```python
from build123d import *

# Parameters (mm, degrees)
SKETCH1_R           = 3.55
SKETCH1_R_2         = 1.5
BOSS_EXTRUDE1_DEPTH = 3


with BuildPart() as part:
    # Sketch1 → Boss-Extrude1 (new body)
    with BuildSketch(Plane.XY):
        with BuildLine():
            Line((4, 0), (4, 9.527864045))
            ThreePointArc((4, 9.527864045), (6, 14), (4, 18.472135955))
            Line((4, 18.472135955), (4, 49))
            ThreePointArc((4, 49), (0, 53), (-4, 49))
            Line((-4, 49), (-4, 18.472135955))
            ThreePointArc((-4, 18.472135955), (-6, 14), (-4, 9.527864045))
            Line((-4, 9.527864045), (-4, 0))
            ThreePointArc((-4, 0), (0, -4), (4, 0))
        make_face()
        with Locations((0, 14)):
            Circle(SKETCH1_R, mode=Mode.SUBTRACT)
        with Locations((0, 49)):
            Circle(SKETCH1_R_2, mode=Mode.SUBTRACT)
        with BuildLine():
            Line((-1, 0), (-1, 5))
            ThreePointArc((-1, 5), (0, 6), (1, 5))
            Line((1, 5), (1, 0))
            ThreePointArc((1, 0), (0, -1), (-1, 0))
        make_face(mode=Mode.SUBTRACT)
        with BuildLine():
            Line((-1, 28), (-1, 23))
            ThreePointArc((-1, 23), (0, 22), (1, 23))
            Line((1, 23), (1, 28))
            ThreePointArc((1, 28), (0, 29), (-1, 28))
        make_face(mode=Mode.SUBTRACT)
    extrude(amount=BOSS_EXTRUDE1_DEPTH)


solid = part.part
```
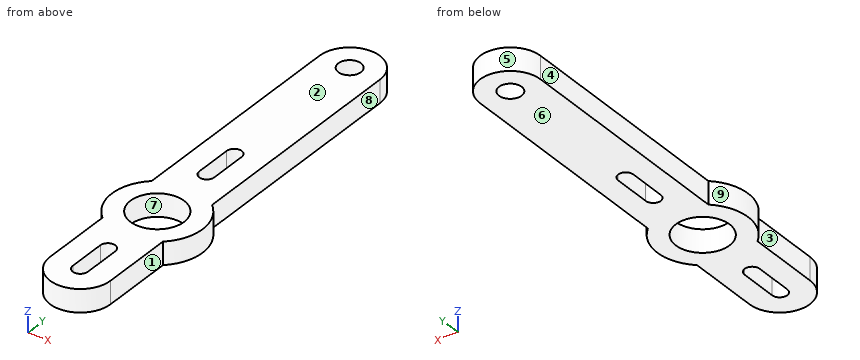
Verification items for the finished model (mm, model axes). Face numbers are marked on the shaded views. A direction names the side the tool comes from. Round coordinates to 2 decimals unless told otherwise and drop trailing zeros. Order: outer loops, then holes, each group sorted by start corner. A loop starts at its lowest first (then second) coordinate and runs counter-clockwise, first axis right, second up.
1) Cross-section at A-A, the plane y = 24. Record the cut outline in (x, z).
Geometry says:
outline: (-4, 0) - (-1, 0) - (-1, 3) - (-4, 3) - close; (1, 0) - (4, 0) - (4, 3) - (1, 3) - close
2) Cross-section at D-D, the plane y = 16. Record the cut outline in (x, z).
Geometry says:
outline: (-5.66, 0) - (-2.93, 0) - (-2.93, 3) - (-5.66, 3) - close; (2.93, 0) - (5.66, 0) - (5.66, 3) - (2.93, 3) - close
3) Cross-section at C-C, the plane x = 0. Record the cut outline in (y, z), plus the area to 3 significant figures.
Geometry says:
outline: (-4, 0) - (-1, 0) - (-1, 3) - (-4, 3) - close; (6, 0) - (10.45, 0) - (10.45, 3) - (6, 3) - close; (17.55, 0) - (22, 0) - (22, 3) - (17.55, 3) - close; (29, 0) - (47.5, 0) - (47.5, 3) - (29, 3) - close; (50.5, 0) - (53, 0) - (53, 3) - (50.5, 3) - close
area: 98.7 mm2
4) Cross-section at B-B, the plane z = 2.4. Record the cut outline in (x, y), plus the area to 3 significant figures.
Geometry says:
outline: (-4, 0) arc R4 ccw to (4, 0) - (4, 9.53) arc R6 ccw to (4, 18.47) - (4, 49) arc R4 ccw to (-4, 49) - (-4, 18.47) arc R6 ccw to (-4, 9.53) - close; hole circle Ø7.1 at (0, 14); hole circle Ø3 at (0, 49); hole (-1, 0) arc R1 ccw to (1, 0) - (1, 5) arc R1 ccw to (-1, 5) - close; hole (-1, 23) arc R1 ccw to (1, 23) - (1, 28) arc R1 ccw to (-1, 28) - close
area: 394 mm2
5) Material ranges on line 1 (Y direction, x = 0, z = 1.4); line 2 (Y direction, x = -0.5, z = 0.9); line 3 (X direction, y = 20, z = 0.25), recorded low to high.
Geometry says:
line 1: y = -4 to -1, 6 to 10.45, 17.55 to 22, 29 to 47.5, 50.5 to 53
line 2: y = -3.97 to -0.87, 5.87 to 10.49, 17.51 to 22.13, 28.87 to 47.59, 50.41 to 52.97
line 3: x = -4 to 4
6) Tool access check on the marked faces 1, 2, 3, 4 and 5. Record the directions out of +Z, -Z, +X, -X, +Y, -Y that give a thin tool (end or side, any length) a straight path to the whole face; none if there is none.
Geometry says:
face 1: +Z, -Z, +X, -Y
face 2: +Z, +X, -X, +Y, -Y
face 3: +Z, -Z, -X, -Y
face 4: +Z, -Z, -X, +Y
face 5: +Z, -Z, +Y
7) Depth check by flat-ended pin: pin 1 (1.5 mm diameter, centred on y = 25.5, z = 2, fed in from +X); pin 2 (1 mm diameter, centred on y = 47, z = 1.5, fed in from -X). Enter the tip coordinate at first touch or a pass-through.
Geometry says:
pin 1: stops at x = 4
pin 2: stops at x = -4
8) Draft check along X on the marked faces 6, 7, 8 and 9. Enter one of: +X half, -X half, draft (parallel to the pull), parting line (faces both ways), or undercut.
Geometry says:
face 6: draft
face 7: undercut
face 8: +X half
face 9: -X half
